Read the model definition and answer for the solid it produces. Units are mm, in the model's axes. A direction names the side the tool comes from. Coordinates: 2 decimals unless noted, no trailing zeros. Loops run counter-clockwise (first coordinate to the right, second up) from the corner with the lowest first, then second, coordinate; pieces in that order, holes last. Notation, with made-up numbers: M -16.75,64.25 L 16.25,64.25 A26 ccw 16.25,83.25 Z; hole C 40.5,16.25 d3. An arc over 180 degrees is marked long. Put each result on its own line as item: value.
from build123d import *

# Parameters (mm, degrees)
SKETCH_1_R          = 20
SKETCH_1_R_2        = 10.5
EXTRUDE_1_DEPTH     = 5
EXTRUDE_START       = -5
EXTRUDE_2_DEPTH     = 5
FILLET_1_R          = 5
SKETCH_3_R          = 2.1
CUT_EXTRUDE_1_DEPTH = 45.582524906
CUT_EXTRUDE_2_DEPTH = 45.582524906
FILLET_2_R          = 2


with BuildPart() as part:
    # 草图1 → 凸台-拉伸1 (new body)
    with BuildSketch(Plane.XY):
        Circle(SKETCH_1_R)
        Circle(SKETCH_1_R_2, mode=Mode.SUBTRACT)
    extrude(amount=EXTRUDE_1_DEPTH)

    # 草图2 → 凸台-拉伸2 (add)
    with BuildSketch(Plane.XY.offset(5).offset(EXTRUDE_START)):
        with BuildLine():
            Line((-28.415563483, -35), (28.415563483, -35))
            Line((28.415563483, -35), (19.580039782, 4.077013874))
            ThreePointArc((19.580039782, 4.077013874), (19.894732917, 2.049293093), (20, 0))
            ThreePointArc((20, 0), (-2.049293093, -19.894732917), (-19.580039782, 4.077013874))
            Line((-19.580039782, 4.077013874), (-28.415563483, -35))
        make_face()
    extrude(amount=EXTRUDE_2_DEPTH)

    # 圆角1
    fillet_1_edges = [part.edges().sort_by_distance(p)[0] for p in [
        (28.415563483, -35, 2.5),
        (-28.415563483, -35, 2.5),
    ]]
    fillet(fillet_1_edges, radius=FILLET_1_R)

    # 草图3 → 切除-拉伸1 (cut, through all)
    with BuildSketch(Plane.XY.offset(5)):
        with Locations((22.158820427, -30)):
            Circle(SKETCH_3_R)
        with Locations((-22.158820427, -30)):
            Circle(SKETCH_3_R)
        with Locations((-18.850745921, -15.36932527)):
            Circle(SKETCH_3_R)
        with Locations((18.850745921, -15.36932527)):
            Circle(SKETCH_3_R)
        Polygon((-16.453332464, -18.36932527), (16.453332464, -18.36932527), (18.404774593, -27), (-18.404774593, -27), align=None)
    extrude(amount=-CUT_EXTRUDE_1_DEPTH, mode=Mode.SUBTRACT)

    # 草图4 → 切除-拉伸2 (cut, through all)
    with BuildSketch(Plane.XY.offset(5)):
        with BuildLine():
            Line((-2.103165657, 10.287210225), (-1.493384576, 11.343382038))
            Line((-1.493384576, 11.343382038), (-8.331863171, 18.181860633))
            ThreePointArc((-8.331863171, 18.181860633), (-14.142135624, 14.142135624), (-18.181860633, 8.331863171))
            Line((-18.181860633, 8.331863171), (-10.481021364, 0.631023902))
            ThreePointArc((-10.481021364, 0.631023902), (-7.931010296, 6.881066464), (-2.103165657, 10.287210225))
        make_face()
        with BuildLine():
            Line((-8.331863171, 18.181860633), (-1.493384576, 11.343382038))
            Line((-1.493384576, 11.343382038), (3.342150011, 19.718773626))
            ThreePointArc((3.342150011, 19.718773626), (-2.610523844, 19.828897227), (-8.331863171, 18.181860633))
        make_face()
        with BuildLine():
            ThreePointArc((-2.103165657, 10.287210225), (-1.370525018, 10.410171044), (-0.631023902, 10.481021364))
            Line((-0.631023902, 10.481021364), (-1.493384576, 11.343382038))
            Line((-1.493384576, 11.343382038), (-2.103165657, 10.287210225))
        make_face()
        with BuildLine():
            Line((-1.493384576, 11.343382038), (-0.631023902, 10.481021364))
            ThreePointArc((-0.631023902, 10.481021364), (5.879816622, 8.699296321), (9.960568218, 3.322210225))
            Line((9.960568218, 3.322210225), (15.405883886, 12.753773626))
            ThreePointArc((15.405883886, 12.753773626), (10, 17.320508076), (3.342150011, 19.718773626))
            Line((3.342150011, 19.718773626), (-1.493384576, 11.343382038))
        make_face()
    extrude(amount=-CUT_EXTRUDE_2_DEPTH, mode=Mode.SUBTRACT)

    # 圆角2
    fillet_2_edges = [part.edges().sort_by_distance(p)[0] for p in [
        (-19.580039782, 4.077013874, 2.5),
        (19.580039782, 4.077013874, 2.5),
        (-18.404774593, -27, 2.5),
        (-16.453332464, -18.36932527, 2.5),
        (16.453332464, -18.36932527, 2.5),
        (18.404774593, -27, 2.5),
        (9.960568218, 3.322210225, 2.5),
        (-10.481021364, 0.631023902, 2.5),
        (-18.181860633, 8.331863171, 2.5),
        (15.405883886, 12.753773626, 2.5),
    ]]
    fillet(fillet_2_edges, radius=FILLET_2_R)


solid = part.part
1) Find section B-B, the plane x = 0. Write down the section's boundary in (y, z), plus the area to 3 significant figures.
Answer list:
outline: M -35,0 L -27,0 L -27,5 L -35,5 Z; M -18.37,0 L -10.5,0 L -10.5,5 L -18.37,5 Z
area: 79.3 mm^2
2) Determine the mould class of faces 1 (the flat face through (0, -35, 2)), 2 (the cylindrical face through (-19.45, 4.66, 2.46)), 3 (the cylindrical face through (-16.91, -16.17, 2.54)), 4 (the flat face through (-13.56, 3.71, 2.54)) for opening direction X: released by +X, released by -X, zero draft, split by the parting line, or undercut.
Answer list:
face 1: zero draft
face 2: released by -X
face 3: undercut
face 4: undercut
3) Find section C-C, the plane z = 1.95. Write down the section's boundary in (x, y), plus the area to 3 significant figures.
Answer list:
outline: M -27.04,-28.9 A5 ccw -22.16,-35 L 22.16,-35 A5 ccw 27.04,-28.9 L 19.58,4.08 A20 ccw 17.3,10.04 A2 ccw 13.84,10.03 L 10.39,4.06 A2 ccw 10.18,2.57 A10.5 cw long -10.5,-0.15 A2 ccw -11.08,1.23 L -15.96,6.11 A2 ccw -19.31,5.22 A20 ccw -19.58,4.08 Z; hole C -22.16,-30 d4.2; hole C -18.85,-15.37 d4.2; hole M -17.85,-24.56 A2 ccw -15.9,-27 L 15.9,-27 A2 ccw 17.85,-24.56 L 16.81,-19.93 A2 ccw 14.86,-18.37 L -14.86,-18.37 A2 ccw -16.81,-19.93 Z; hole C 18.85,-15.37 d4.2; hole C 22.16,-30 d4.2
area: 1,290 mm^2
4) Which of the six approach directions +Z, -Z, +X, -X, +Y, -Y give full straight-line access (tool end or side, diameter ignored) to faces 5 (the cylindrical face through (18.694, 7.108, 2.465)), 6 (the flat face through (0, -18.369, 3))?
Answer list:
face 5: +Z, -Z, +X, +Y
face 6: +Z, -Z
5) Straight lines are drawn through the part: line 1 (Y direction, x = 0, z = 1.3); line 2 (X direction, y = -14, z = 4.15); line 3 (Y direction, x = 9, z = 3.4). For each, find the intervals that lie inside material, in ascending order. Write a range as [from, to].
Answer list:
line 1: y = [-35, -27], [-18.37, -10.5]
line 2: x = [-23.67, -20.44], [-17.26, 17.26], [20.44, 23.67]
line 3: y = [-35, -27], [-18.37, -5.41]
6) Given pin 1 Ø1.5 at (x, z) = (-2, 2.5) entering from +Y; pin 2 Ø1 at (x, z) = (17.5, 1) entering from +Y; pin 3 Ø2 at (y, z) = (2, 2.5) entering from -X; pin 4 Ø17 at (x, y) = (0, 0) entering from -Z, each flat-ended and moving along its own axis, determine where each tip first touches the part or whether it passes through.
Answer list:
pin 1: stops at y = -10.13
pin 2: stops at y = 10.43
pin 3: stops at x = -20.28
pin 4: passes through
7) Find section D-D, the plane y = -9. Write down the section's boundary in (x, z).
Answer list:
outline: M -22.54,0 L -5.41,0 L -5.41,5 L -22.54,5 Z; M 5.41,0 L 22.54,0 L 22.54,5 L 5.41,5 Z
8) Find section A-A, the plane y = -30. Write down the section's boundary in (x, z).
Answer list:
outline: M -27.16,0 L -24.26,0 L -24.26,5 L -27.16,5 Z; M -20.06,0 L 20.06,0 L 20.06,5 L -20.06,5 Z; M 24.26,0 L 27.16,0 L 27.16,5 L 24.26,5 Z
